Answer from the drawing. Dimensions are ordinates in mm from the lowest x, y and z of the part. A direction names the side the tool comes from. Coordinates: 2 decimals unless noted, no trailing zeros. Order: outer loops, then holes, each group sorted by start corner. A loop starts at its lowest first (then second) coordinate and runs counter-clockwise, first axis right, second up. Notation, with made-up numbers: (19, 48.25) -> (61, 48.25) arc R13 ccw to (61, 71.25) -> close; hole circle Ø6 at (73.25, 36.25). An arc over 180 degrees is marked (long way). Answer in a Markdown table with one row per item.
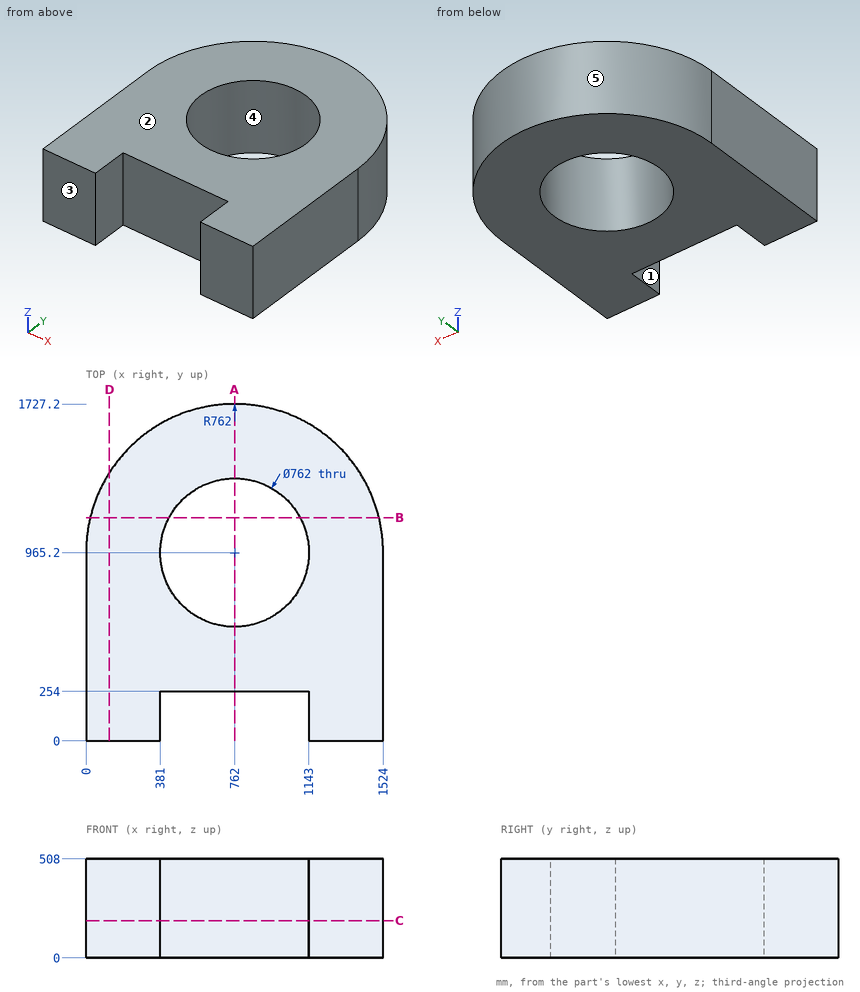
(1) Find the intervals of material crossed by line 1 along Y through (x, z) = (762, 179); line 2 along X through (y, z) = (965, 148); line 3 along X through (y, z) = (958, 125), in increasing order. Write a range as from..to.
Check values:
| item | result |
|---|---|
| line 1 | 254..584.2, 1346.2..1727.2 |
| line 2 | 0..381, 1143..1524 |
| line 3 | 0..381.07, 1142.93..1524 |
(2) A cutting plane is placed at B-B, the plane y = 1145. Determine the outline of the cut face in (x, z).
Check values:
| item | result |
|---|---|
| outline | (21.52, 0) -> (426.09, 0) -> (426.09, 508) -> (21.52, 508) -> close; (1097.91, 0) -> (1502.48, 0) -> (1502.48, 508) -> (1097.91, 508) -> close |
(3) A cutting plane is placed at C-C, the plane z = 191. Determine the outline of the cut face in (x, y), then the cut area to 3 significant figures.
Check values:
| item | result |
|---|---|
| outline | (0, 0) -> (381, 0) -> (381, 254) -> (1143, 254) -> (1143, 0) -> (1524, 0) -> (1524, 965.2) arc R762 ccw to (0, 965.2) -> close; hole circle Ø762 at (762, 965.2) |
| area | 1,730,000 mm² |
(4) A cutting plane is placed at A-A, the plane x = 762. Determine the outline of the cut face in (y, z).
Check values:
| item | result |
|---|---|
| outline | (254, 0) -> (584.2, 0) -> (584.2, 508) -> (254, 508) -> close; (1346.2, 0) -> (1727.2, 0) -> (1727.2, 508) -> (1346.2, 508) -> close |
(5) For a pull along X with two mould halves and no side action, classify the marked faces 3, 4 and 5 as released by +X, released by -X, zero draft, split by the parting line, or undercut.
Check values:
| item | result |
|---|---|
| face 3 | zero draft |
| face 4 | undercut |
| face 5 | split by the parting line |
(6) A cutting plane is placed at D-D, the plane x = 120.5. Determine the outline of the cut face in (y, z).
Check values:
| item | result |
|---|---|
| outline | (0, 0) -> (1376.44, 0) -> (1376.44, 508) -> (0, 508) -> close |
(7) Which of the six approach directions +Z, -Z, +X, -X, +Y, -Y give full straight-line access (tool end or side, diameter ignored) to the marked faces 1 and 2?
Check values:
| item | result |
|---|---|
| face 1 | +Z, -Z, -Y |
| face 2 | +Z, +X, -X, +Y, -Y |
(8) Flat-ended cylindrical pins translate along their axes: pin 1 (12 mm diameter, centred on x = 551, z = 130.5, fed in from +Y); pin 2 (1 mm diameter, centred on y = 1265.5, z = 320, fed in from -X); pin 3 (4 mm diameter, centred on x = 349.5, y = 279, fed in from -Z). Find the tip coordinate at first contact, or state that the pin passes through.
Check values:
| item | result |
|---|---|
| pin 1 | y = 1699.11 |
| pin 2 | x = 61.45 |
| pin 3 | z = 0 |
